Answer from the drawing. Dimensions are ordinates in mm from the lowest x, y and z of the part. Round coordinates to 2 decimals unless told otherwise and drop trailing zeros. Order: outer loops, then holes, each group sorted by start corner. A loop starts at its lowest first (then second) coordinate and runs counter-clockwise, first axis right, second up.
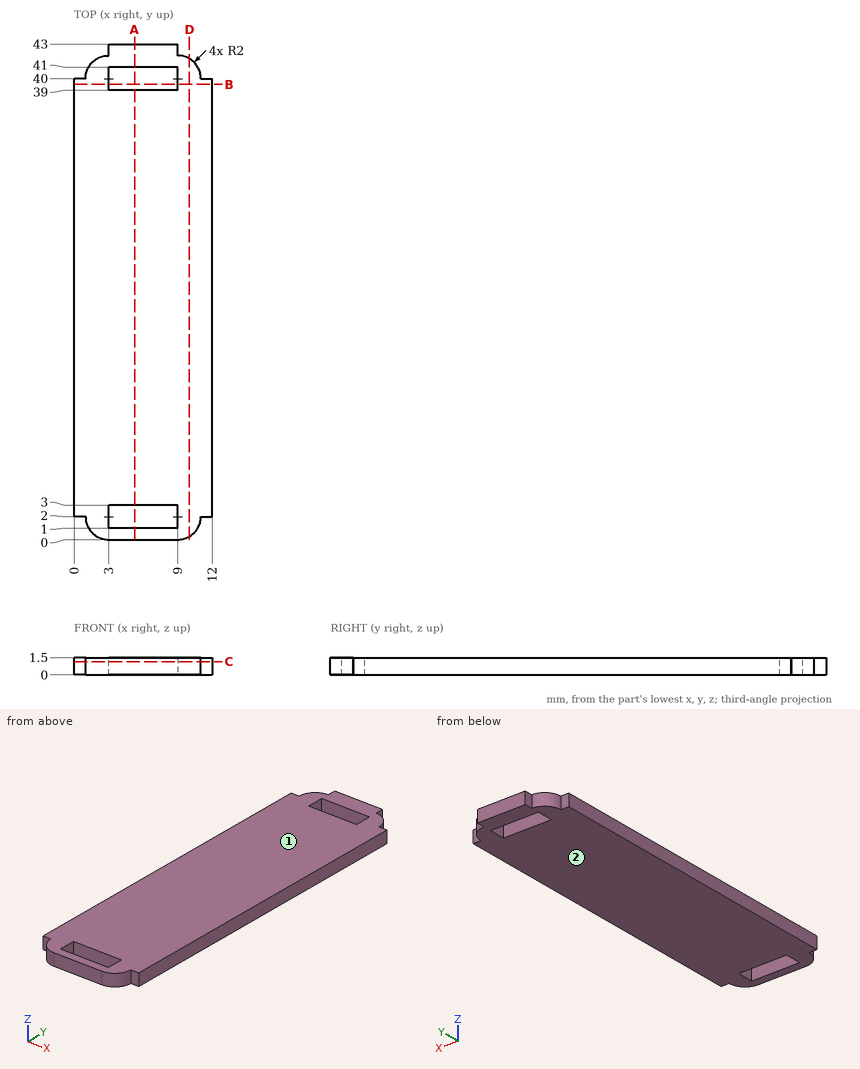
Q1. Straight lines are drawn through the part: probe 1 along Y at (x, z) = (6, 1.1); probe 2 along Y at (x, z) = (11.5, 1.3); probe 3 along Y at (x, z) = (10.25, 0.65). For each, find the intervals that lie inside material, in ascending order.
Outcome:
probe 1: y = 0 to 1, 3 to 39, 41 to 43
probe 2: y = 2 to 40
probe 3: y = 0.44 to 41.56
Q2. Flat-ended cylindrical pins translate along their axes: pin 1 (0.8 mm diameter, centred on y = 42.5, z = 1, fed in from +X); pin 2 (5 mm diameter, centred on x = 9, y = 17, fed in from -Z); pin 3 (0.5 mm diameter, centred on x = 0.5, z = 1, fed in from -Y). Find the tip coordinate at first contact, or state that the pin passes through.
Outcome:
pin 1: stops at x = 9
pin 2: stops at z = 0
pin 3: stops at y = 2
Q3. A cutting plane is placed at D-D, the plane x = 10. Give the vertices of the cut face in (y, z).
Outcome:
outline: (0.27, 0) - (41.73, 0) - (41.73, 1.5) - (0.27, 1.5) - close
Q4. For a pull along Z with two mould halves and no side action, classify the marked faces 1 and 2 as released by +Z, released by -Z, zero draft, split by the parting line, or undercut.
Outcome:
face 1: released by +Z
face 2: released by -Z
Q5. A cutting plane is placed at A-A, the plane x = 5.25. Give the vertices of the cut face in (y, z), plus the area to 3 significant figures.
Outcome:
outline: (0, 0) - (1, 0) - (1, 1.5) - (0, 1.5) - close; (3, 0) - (39, 0) - (39, 1.5) - (3, 1.5) - close; (41, 0) - (43, 0) - (43, 1.5) - (41, 1.5) - close
area: 58.5 mm2
Q6. A cutting plane is placed at B-B, the plane y = 39.5. Give the vertices of the cut face in (x, z).
Outcome:
outline: (0, 0) - (3, 0) - (3, 1.5) - (0, 1.5) - close; (9, 0) - (12, 0) - (12, 1.5) - (9, 1.5) - close
Q7. A cutting plane is placed at C-C, the plane z = 1.15. Give the vertices of the cut face in (x, y), plus the area to 3 significant figures.
Outcome:
outline: (0, 2) - (1, 2) arc R2 ccw to (3, 0) - (9, 0) arc R2 ccw to (11, 2) - (12, 2) - (12, 40) - (11, 40) arc R2 ccw to (9, 42) - (9, 43) - (3, 43) - (3, 42) arc R2 ccw to (1, 40) - (0, 40) - close; hole (3, 1) - (9, 1) - (9, 3) - (3, 3) - close; hole (3, 39) - (9, 39) - (9, 41) - (3, 41) - close
area: 475 mm2
